Geometry check sheet. Reference: drawing and pictorial views, mm from the part's lowest x, y, z. A direction names the side the tool comes from. Give positions to 0.01 mm unless a question says otherwise; leave off trailing zeros. Write each loop counter-clockwise with the first axis right and the second up, starting at its lowest first coordinate (ties: lowest second). Pieces come first, ordered by that corner, then holes. Notation, with made-up numbers: (12, -26.75) - (49, -26.75) arc R23 cw to (49, -16.75) - close; hole circle Ø5 at (8, -26.75). An arc over 180 degrees is marked (long way). Put each result on its own line as item: value.
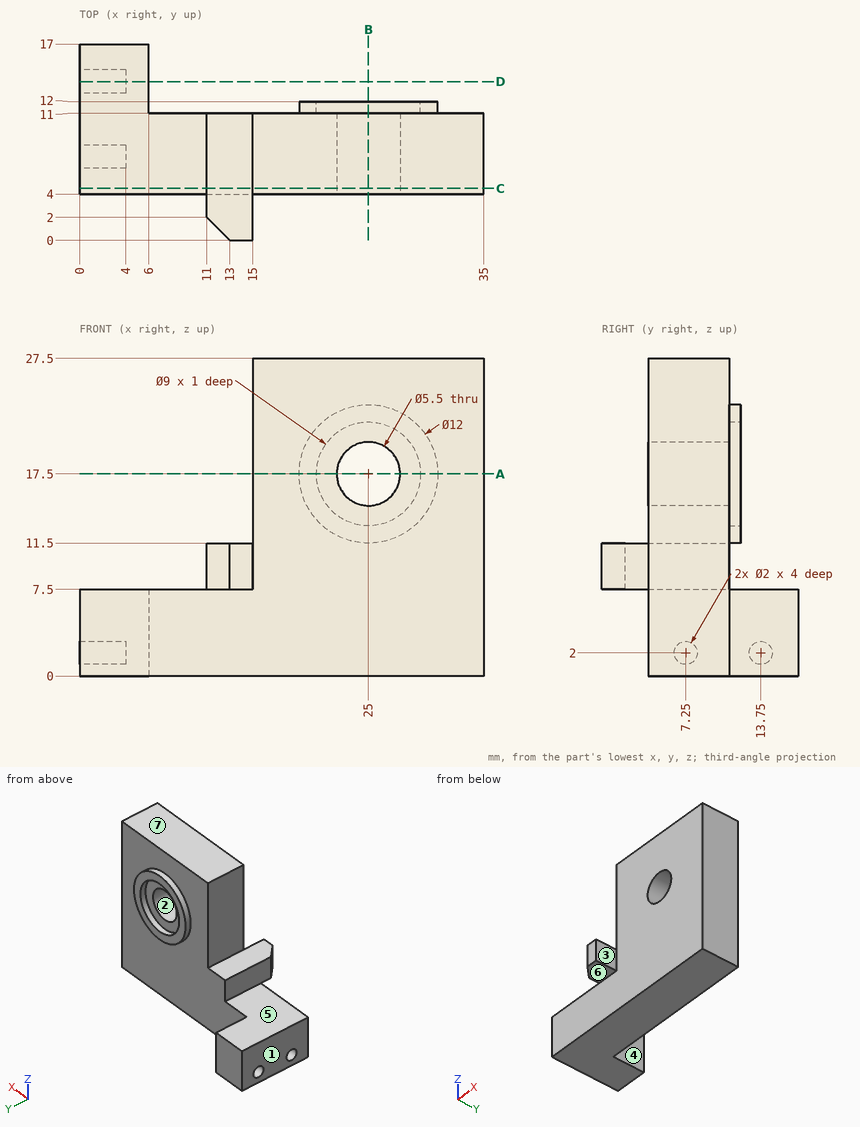
Q1. Go/stop test with flat-tipped pins: pin 1 Ø9.5 at (x, z) = (27.5, 17.5) entering from +Y; pin 2 Ø2 at (x, y) = (12.5, 3) entering from +Z; pin 3 Ø3 at (x, y) = (5.5, 7) entering from +Z; pin 4 Ø2.5 at (x, z) = (25.5, 17.5) entering from +Y. Record where each tip stops, or that it passes through.
Answers follow:
pin 1: stops at y = 12
pin 2: stops at z = 11.5
pin 3: stops at z = 7.5
pin 4: passes through
Q2. Section check C-C, the plane y = 4.5. Record the cut outline in (x, z).
Answers follow:
outline: (0, 0) - (35, 0) - (35, 27.5) - (15, 27.5) - (15, 11.5) - (11, 11.5) - (11, 7.5) - (0, 7.5) - close; hole circle Ø5.5 at (25, 17.5)
Q3. Section check A-A, the plane z = 17.5. Record the cut outline in (x, y).
Answers follow:
outline: (15, 4) - (22.25, 4) - (22.25, 11) - (20.5, 11) - (20.5, 12) - (19, 12) - (19, 11) - (15, 11) - close; (27.75, 4) - (35, 4) - (35, 11) - (31, 11) - (31, 12) - (29.5, 12) - (29.5, 11) - (27.75, 11) - close
Q4. Set-up check for the marked faces 4, 5, 6 and 7: record each of +Z, -Z, +X, -X, +Y, -Y from which the full face is reachable in a straight line by a thin tool's end or side.
Answers follow:
face 4: +Z, -Z, +X, +Y
face 5: +Z, -X, +Y, -Y
face 6: -Z, +X, -X, -Y
face 7: +Z, +X, -X, +Y, -Y
Q5. Release check for a two-part mould opening along X. For the marked faces 1, 2 and 3 record: released by +X, released by -X, zero draft, split by the parting line, or undercut.
Answers follow:
face 1: released by -X
face 2: undercut
face 3: released by +X
Q6. Section check D-D, the plane y = 13.75. Record the cut outline in (x, z).
Answers follow:
outline: (0, 0) - (6, 0) - (6, 7.5) - (0, 7.5) - (0, 3) - (4, 3) - (4, 1) - (0, 1) - close
Q7. Scan lines: line 1 along Y through (x, z) = (3.15, 2); line 2 along Z through (x, y) = (25, 6.5); line 3 along X through (y, z) = (9, 17.5). Record each from-to range of solid material in increasing order.
Answers follow:
line 1: y = 4 to 6.25, 8.25 to 12.75, 14.75 to 17
line 2: z = 0 to 14.75, 20.25 to 27.5
line 3: x = 15 to 22.25, 27.75 to 35
Q8. Section check B-B, the plane x = 25. Record the cut outline in (y, z), plus the area to 3 significant figures.
Answers follow:
outline: (4, 0) - (11, 0) - (11, 11.5) - (12, 11.5) - (12, 13) - (11, 13) - (11, 14.75) - (4, 14.75) - close; (4, 20.25) - (11, 20.25) - (11, 22) - (12, 22) - (12, 23.5) - (11, 23.5) - (11, 27.5) - (4, 27.5) - close
area: 157 mm2
